```python
from build123d import *
from build123d.topology import SkipClean

# Parameters (mm, degrees)
BOSS_EXTRUDE1_DEPTH = 10
BOSS_EXTRUDE3_DEPTH = 50
SKETCH3_W           = 18.659519989
SKETCH3_H           = 24
CUT_EXTRUDE2_DEPTH  = 16
SKETCH4_W           = 7.007010428
SKETCH4_H           = 3.464986189
CUT_EXTRUDE4_DEPTH  = 11
SKETCH6_R           = 1.75
CUT_EXTRUDE5_DEPTH  = 50
SKETCH7_R           = 1.1
CUT_EXTRUDE6_DEPTH  = 10
SKETCH8_R           = 1.1
CUT_EXTRUDE7_DEPTH  = 10
SKETCH12_R          = 1.75
CUT_EXTRUDE11_DEPTH = 6
SKETCH13_R          = 1.75
CUT_EXTRUDE12_DEPTH = 6
CUT_EXTRUDE13_START = -6
SKETCH15_R          = 1.75
CUT_EXTRUDE13_DEPTH = 6
CUT_EXTRUDE14_START = -6
SKETCH16_R          = 1.75
CUT_EXTRUDE14_DEPTH = 6


with BuildPart() as part:
    # Sketch1 → Boss-Extrude1 (new body)
    with BuildSketch(Plane(origin=(0, 0, 0), x_dir=(1, 0, 0), z_dir=(0, 1, 0))):
        with BuildLine():
            Line((-20.369908508, -22.9), (20.369908508, -22.9))
            Line((20.369908508, -22.9), (25.75194079, -25.156262551))
            ThreePointArc((25.75194079, -25.156262551), (36, 0), (25.75194079, 25.156262551))
            Line((25.75194079, 25.156262551), (20.369908508, 22.9))
            Line((20.369908508, 22.9), (-20.369908508, 22.9))
            Line((-20.369908508, 22.9), (-25.75194079, 25.156262551))
            ThreePointArc((-25.75194079, 25.156262551), (-30.058427692, 19.811383714), (-33.272198921, 13.746300555))
            Line((-33.272198921, 13.746300555), (-20.930426703, 13.746300555))
            ThreePointArc((-20.930426703, 13.746300555), (-18.911500586, 16.969147591), (-16.488091862, 19.9))
            Line((-16.488091862, 19.9), (16.488091862, 19.9))
            ThreePointArc((16.488091862, 19.9), (24.396538405, 0), (16.488091862, -19.9))
            Line((16.488091862, -19.9), (-16.488091862, -19.9))
            ThreePointArc((-16.488091862, -19.9), (-20.300121646, -14.857351831), (-22.928570874, -9.108340935))
            Line((-22.928570874, -9.108340935), (-34.828696866, -9.108340935))
            ThreePointArc((-34.828696866, -9.108340935), (-31.335081965, -17.723223133), (-25.75194079, -25.156262551))
            Line((-25.75194079, -25.156262551), (-20.369908508, -22.9))
        make_face()
    extrude(amount=BOSS_EXTRUDE1_DEPTH)

    # Sketch1_5 → Boss-Extrude3 (add)
    with BuildSketch(Plane(origin=(0, 0, 0), x_dir=(1, 0, 0), z_dir=(0, 1, 0))):
        with BuildLine():
            ThreePointArc((-33.272198921, 13.746300555), (-35.916801934, 2.44608643), (-34.828696866, -9.108340935))
            Line((-34.828696866, -9.108340935), (-22.928570874, -9.108340935))
            ThreePointArc((-22.928570874, -9.108340935), (-24.286368586, 2.525037107), (-20.930426703, 13.746300555))
            Line((-20.930426703, 13.746300555), (-33.272198921, 13.746300555))
        make_face()
    extrude(amount=BOSS_EXTRUDE3_DEPTH)

    # Sketch3 → Cut-Extrude2 (cut)
    with BuildSketch(Plane.XY.offset(9.108340935)):
        with Locations((-32.258330869, 27)):
            Rectangle(SKETCH3_W, SKETCH3_H)
    extrude(amount=-CUT_EXTRUDE2_DEPTH, mode=Mode.SUBTRACT)

    # Sketch4 → Cut-Extrude4 (cut)
    with BuildSketch(Plane(origin=(0, 50, 0), x_dir=(1, 0, 0), z_dir=(0, 1, 0))):
        with Locations((-27.295412644, 1.732493095)):
            Rectangle(SKETCH4_W, SKETCH4_H)
    extrude(amount=-CUT_EXTRUDE4_DEPTH, mode=Mode.SUBTRACT)

    # Sketch6 → Cut-Extrude5 (cut)
    with BuildSketch(Plane(origin=(0, 0, -22.9), x_dir=(-1, 0, 0), z_dir=(0, 0, -1))):
        with Locations((0, 5.25)):
            Circle(SKETCH6_R)
    extrude(amount=-CUT_EXTRUDE5_DEPTH, mode=Mode.SUBTRACT)

    # Sketch7 → Cut-Extrude6 (cut)
    with BuildSketch(Plane.XY.offset(9.108340935)):
        with Locations((-28.103908, 40.912886193)):
            Circle(SKETCH7_R)
    extrude(amount=-CUT_EXTRUDE6_DEPTH, mode=Mode.SUBTRACT)

    # Sketch8 → Cut-Extrude7 (cut)
    with BuildSketch(Plane.XY.offset(9.108340935)):
        with Locations((-27.944858765, 13.113341173)):
            Circle(SKETCH8_R)
    extrude(amount=-CUT_EXTRUDE7_DEPTH, mode=Mode.SUBTRACT)

    # Sketch12 → Cut-Extrude11 (cut)
    with BuildSketch(Plane(origin=(30.999475006, 10, 18.303894377), x_dir=(0.5084415104778145, 0, -0.8610965279357702), z_dir=(0.8610965279357702, 0, 0.5084415104778145))):
        with Locations((0, -5)):
            Circle(SKETCH12_R)
    extrude(amount=-CUT_EXTRUDE11_DEPTH, mode=Mode.SUBTRACT)

    # Sketch13 → Cut-Extrude12 (cut)
    with BuildSketch(Plane(origin=(30.999475006, 10, -18.303894377), x_dir=(-0.5084415104778145, 0, -0.8610965279357701), z_dir=(0.8610965279357701, 0, -0.5084415104778145))):
        with Locations((0, -5)):
            Circle(SKETCH13_R)
    extrude(amount=-CUT_EXTRUDE12_DEPTH, mode=Mode.SUBTRACT)

    # Sketch15 → Cut-Extrude13 (cut)
    with SkipClean():  # the faces are left unmerged after this step: merging them gives an invalid solid
        with BuildSketch(Plane(origin=(-30.999475006, 10, 18.303894377), x_dir=(0.5084415104778142, 0, 0.8610965279357703), z_dir=(-0.8610965279357703, 0, 0.5084415104778142)).offset(CUT_EXTRUDE13_START)):
            with Locations(Location((0, -5, 0), (0, 0, 180))):
                Circle(SKETCH15_R)
        extrude(amount=CUT_EXTRUDE13_DEPTH, mode=Mode.SUBTRACT)

    # Sketch16 → Cut-Extrude14 (cut)
    with SkipClean():  # the faces are left unmerged after this step: merging them gives an invalid solid
        with BuildSketch(Plane(origin=(-30.999475006, 10, -18.303894377), x_dir=(-0.508441510477814, 0, 0.8610965279357704), z_dir=(-0.8610965279357704, 0, -0.508441510477814)).offset(CUT_EXTRUDE14_START)):
            with Locations(Location((0, -5, 0), (0, 0, 180))):
                Circle(SKETCH16_R)
        extrude(amount=CUT_EXTRUDE14_DEPTH, mode=Mode.SUBTRACT)


solid = part.part
```
Input: part model. Units: mm. Frame: model coordinates. A direction names the side the tool comes from. Round coordinates to 2 decimals unless told otherwise and drop trailing zeros. Loops run counter-clockwise (first coordinate to the right, second up) from the corner with the lowest first, then second, coordinate; pieces in that order, holes last. Notation, with made-up numbers: (16.5, 74.25) - (25.5, 74.25) arc R16 cw to (25.5, 82.25) - close; hole circle Ø7 at (12.5, 46). An arc over 180 degrees is marked (long way). One line per item, written item: value. Start each with the question number.
(1) Ray query, line 1 (Y direction, x = 0, z = 20.95); line 2 (Y direction, x = -30, z = 7.5); line 3 (Z direction, x = -26, y = 24). Return the intervals inside material, ascending. Write a range as [from, to].
(2) Draft query along Z for faces 1 (the flat face through (-27, 30, -13.746)), 2 (the flat face through (-25.845, 4.976, -15.232)), 3 (the flat face through (-28, 13, -0.892)). Return one class per face: +Z half, -Z half, draft (parallel to the pull), parting line (faces both ways), or undercut.
(3) Access query for faces 4 (the flat face through (-28, 45, -3.465)), 5 (the cylindrical face through (-24.017, 44.423, 4.677)), 6 (the flat face through (0, 3, -19.9)). Directions: +Z, -Z, +X, -X, +Y, -Y. A direction counts if a zero-diameter tool reaches every point of the face in a straight line with its end or side. Return the directions, or none.
(4) Section A-A, the plane x = -10.5. Return loops of the section in (y, z).
(5) Contact query for flat-ended pins moving along their axis: P1, Ø6, axis at x = -23.5, z = 16, coming from the +Y side; P2, Ø6, axis at x = -29, y = 28, coming from the +Z side; P3, Ø12, axis at y = 6, z = -16.5, coming from the +X side. Output: stop coordinate, or through.
(6) Section B-B, the plane y = 9. Return loops of the section in (x, z), plus the area to 3 significant figures.
(7) Section D-D, the plane z = 21.5. Return loops of the section in (x, y), plus the area to 3 significant figures.
(8) Section C-C, the plane x = 0. Return loops of the section in (y, z).
Results below:
1. line 1: [0, 3.5], [7, 10]
1. line 2: [0, 15], [39, 50]
1. line 3: [-13.75, -6.89]
2. face 1: -Z half
2. face 2: undercut
2. face 3: +Z half
3. face 4: +X, +Y
3. face 5: +X, +Y, -Y
3. face 6: +Y, -Y
4. outline: (0, -22.9) - (10, -22.9) - (10, -19.9) - (0, -19.9) - close; (0, 19.9) - (10, 19.9) - (10, 22.9) - (0, 22.9) - close
5. P1: y = 10
5. P2: z = -6.89
5. P3: x = 34.43
6. outline: (-25.75, -25.16) - (-20.37, -22.9) - (20.37, -22.9) - (25.75, -25.16) arc R36 ccw to (25.75, 25.16) - (20.37, 22.9) - (-20.37, 22.9) - (-25.75, 25.16) arc R36 ccw to start; hole (-16.49, -19.9) - (16.49, -19.9) arc R28.99 ccw to (16.49, 19.9) - (-16.49, 19.9) arc R28.99 ccw to start
6. area: 1,350 mm^2
7. outline: (-28.87, 0) - (28.87, 0) - (28.87, 10) - (-28.87, 10) - close; hole circle Ø3.5 at (0, 5.25)
7. area: 568 mm^2
8. outline: (0, -22.9) - (3.5, -22.9) - (3.5, -19.9) - (0, -19.9) - close; (0, 19.9) - (3.5, 19.9) - (3.5, 22.9) - (0, 22.9) - close; (7, -22.9) - (10, -22.9) - (10, -19.9) - (7, -19.9) - close; (7, 19.9) - (10, 19.9) - (10, 22.9) - (7, 22.9) - close
